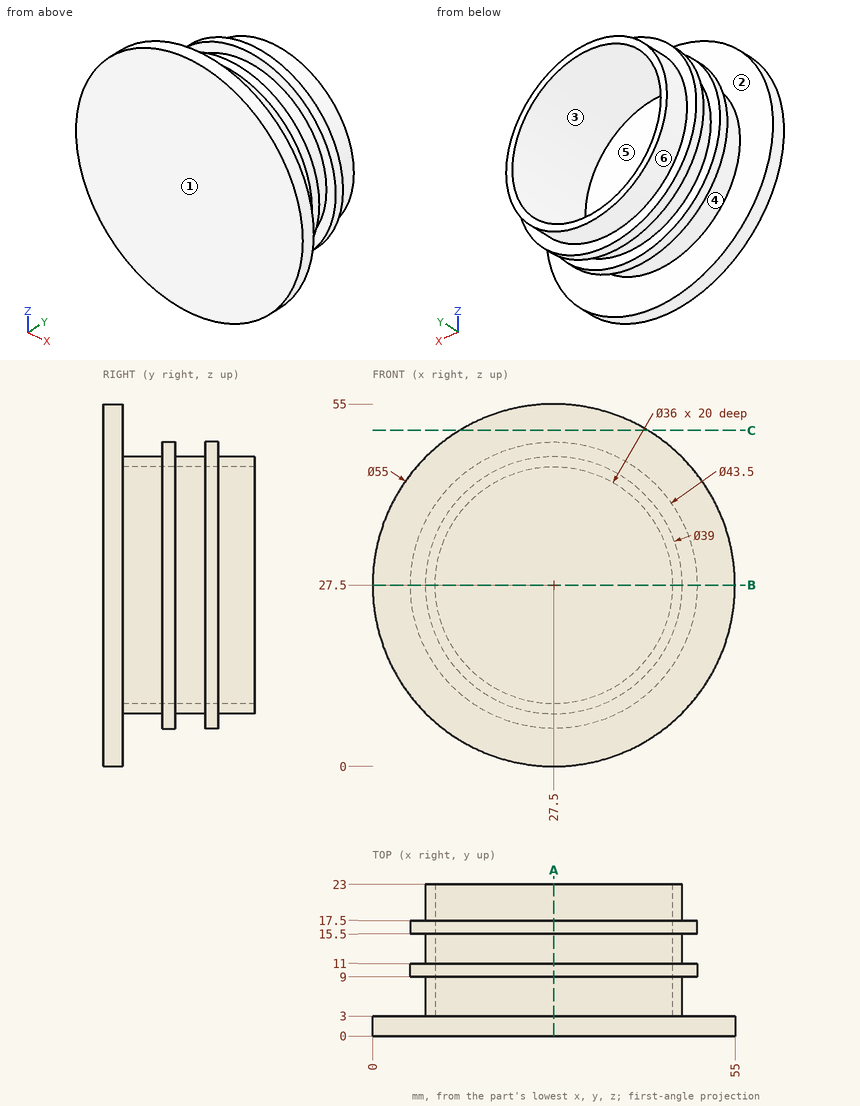
Source: three-view drawing plus pictorial views. Frame: mm from the lowest corner of the part. A direction names the side the tool comes from. Round coordinates to 2 decimals unless told otherwise and drop trailing zeros. Loops run counter-clockwise (first coordinate to the right, second up) from the corner with the lowest first, then second, coordinate; pieces in that order, holes last.
Q1. Section B-B on z = 27.5. Return loops of the section in (x, y).
Q2. Section C-C on z = 51. Return loops of the section in (x, y), plus the area to 3 significant figures.
Q3. Pin query (flat end, axial travel): P1, Ø13, axis at x = 30.5, z = 27.5, coming from the +Y side; P2, Ø5, axis at y = 4, z = 30.5, coming from the -X side; P3, Ø12, axis at x = 28, z = 10, coming from the +Y side; P4, Ø1.5, axis at y = 11, z = 14.5, coming from the +X side. Return the tip coordinate at first contact, or that it passes through.
Q4. Material intervals for L1, parallel to Y at x = 42.5, z = 12.5; L2, parallel to Z at x = 27.5, y = 18.75, sorted ascending.
Q5. Section A-A on x = 27.5. Return loops of the section in (y, z), plus the area to 3 significant figures.
Q6. Access query for the marked faces 1, 2 and 3. Directions: +Z, -Z, +X, -X, +Y, -Y. A direction counts if a zero-diameter tool reaches every point of the face in a straight line with its end or side. Return the directions, or none.
Q7. Pull-direction query (Y, two-part tool) for the marked faces 4, 5 and 6; classes: released by +Y, released by -Y, zero draft, split by the parting line, or undercut.
Evaluation:
1. outline: (0, 0) - (55, 0) - (55, 3) - (47, 3) - (47, 9) - (49.25, 9) - (49.25, 11) - (47, 11) - (47, 15.5) - (49.25, 15.5) - (49.25, 17.5) - (47, 17.5) - (47, 23) - (45.5, 23) - (45.5, 3) - (9.5, 3) - (9.5, 23) - (8, 23) - (8, 17.5) - (5.75, 17.5) - (5.75, 15.5) - (8, 15.5) - (8, 11) - (5.75, 11) - (5.75, 9) - (8, 9) - (8, 3) - (0, 3) - close
2. outline: (13.22, 0) - (41.78, 0) - (41.78, 3) - (13.22, 3) - close
2. area: 85.7 mm2
3. P1: stops at y = 3
3. P2: stops at x = 0.01
3. P3: stops at y = 23
3. P4: stops at x = 45.47
4. L1: y = 0 to 3, 9 to 11, 15.5 to 17.5
4. L2: z = 8 to 9.5, 45.5 to 47
5. outline: (0, 0) - (3, 0) - (3, 8) - (9, 8) - (9, 5.75) - (11, 5.75) - (11, 8) - (15.5, 8) - (15.5, 5.75) - (17.5, 5.75) - (17.5, 8) - (23, 8) - (23, 9.5) - (3, 9.5) - (3, 45.5) - (23, 45.5) - (23, 47) - (17.5, 47) - (17.5, 49.25) - (15.5, 49.25) - (15.5, 47) - (11, 47) - (11, 49.25) - (9, 49.25) - (9, 47) - (3, 47) - (3, 55) - (0, 55) - close
5. area: 243 mm2
6. face 1: +Z, -Z, +X, -X, -Y
6. face 2: none
6. face 3: +Y
7. face 4: undercut
7. face 5: released by +Y
7. face 6: zero draft
